Autodesk Inventor part; units mm, degrees
ref_plane "YZ Plane" through (0, 0, 0) normal (1, 0, 0) x (0, 1, 0)
ref_plane "XZ Plane" through (0, 0, 0) normal (0, 1, 0) x (-1, 0, 0)
ref_plane "XY Plane" through (0, 0, 0) normal (0, 0, 1) x (1, 0, 0)
sketch "Skizze1" plane through (0, 0, 0) normal (0, 1, 0) x (-1, 0, 0)
  line L0 (0, 0) -> (-206, 0)
  line L1 (-206, 0) -> (-206, -100)
  line L2 (-206, -100) -> (0, -100)
  line L3 (0, -100) -> (0, 0)
  dimension "d0" = 206
  dimension "d1" = 100
extrude "Extrusion1" add sketch "Skizze1" along normal blind 10
sketch "Skizze2" plane through (0, 10, 0) normal (0, 1, 0) x (1, 0, 0)
  line L0 (206, 100) -> (0, 100) construction
  line L1 (0, 100) -> (0, 20) construction
  line L2 (0, 100) -> (0, 0) construction
  line L3 (0, 100) -> (80, 100) construction
  line L4 (0, 20) -> (206, 20) construction
  line L5 (206, 20) -> (103, 20) construction
  line L6 (206, 20) -> (309, 20) construction
  line L7 (103, 20) -> (153, 20) construction
  line L8 (103, 20) -> (153, 20) construction
  line L9 (153, 20) -> (147, 20)
  line L10 (147, 20) -> (147, 26)
  line L11 (147, 26) -> (153, 26)
  line L12 (153, 26) -> (153, 20)
  line L13 (147, 20) -> (153, 20)
  line L14 (153, 20) -> (153, 14)
  line L15 (153, 14) -> (147, 14)
  line L16 (147, 14) -> (147, 20)
  arc A0 (147, 14) -> (153, 8) centre (153, 14) ccw
  arc A1 (153, 32) -> (147, 26) centre (153, 26) ccw
  line L17 (153, 8) -> (153, 32)
  line L18 (306, 20) -> (100, 20) construction
  line L19 (100, 20) -> (203, 20) construction
  line L20 (203, 20) -> (153, 20) construction
  line L21 (203, 20) -> (153, 20) construction
  line L22 (153, 20) -> (159, 20)
  line L23 (159, 20) -> (159, 26)
  line L24 (159, 26) -> (153, 26)
  line L25 (159, 20) -> (153, 20)
  line L26 (153, 14) -> (159, 14)
  line L27 (159, 14) -> (159, 20)
  arc A2 (153, 8) -> (159, 14) centre (153, 14) ccw
  arc A3 (159, 26) -> (153, 32) centre (153, 26) ccw
  line L28 (103, 100) -> (103, 20) construction
  line L29 (0, 0) -> (206, 0) construction
  line L30 (103, 100) -> (183, 100) construction
  line L31 (53, 20) -> (59, 20)
  line L32 (59, 20) -> (59, 26)
  line L33 (59, 26) -> (53, 26)
  line L34 (53, 26) -> (53, 20)
  line L35 (59, 20) -> (53, 20)
  line L36 (53, 20) -> (53, 14)
  line L37 (53, 14) -> (59, 14)
  line L38 (59, 14) -> (59, 20)
  arc A4 (53, 8) -> (59, 14) centre (53, 14) ccw
  arc A5 (59, 26) -> (53, 32) centre (53, 26) ccw
  line L39 (53, 8) -> (53, 32)
  line L40 (47, 20) -> (47, 26)
  line L41 (47, 26) -> (53, 26)
  line L42 (53, 20) -> (47, 20)
  line L43 (47, 20) -> (53, 20)
  line L44 (47, 14) -> (47, 20)
  line L45 (53, 14) -> (47, 14)
  arc A6 (53, 32) -> (47, 26) centre (53, 26) ccw
  arc A7 (47, 14) -> (53, 8) centre (53, 14) ccw
  dimension "d4" = 80
  dimension "d5" = 90
  dimension "d6" = 206
  dimension "d7" = 90
  dimension "d8" = 103
  dimension "d9" = 180
  dimension "d10" = 50
  dimension "d11" = 0
  dimension "d12" = 6
  dimension "d13" = 6
  dimension "d14" = 6
  dimension "d15" = 6
  dimension "d16" = 80
  dimension "d17" = 90
extrude "Extrusion2" cut sketch "Skizze2" against normal blind 10
sketch "Skizze4" plane through (0, 10, 0) normal (0, 1, 0) x (1, 0, 0)
  line L0 (0, 100) -> (0, 80) construction
  line L1 (0, 100) -> (0, 0) construction
  line L2 (0, 100) -> (20, 100) construction
  line L3 (0, 80) -> (206, 80) construction
  line L4 (0, 80) -> (103, 80) construction
  line L5 (103, 80) -> (53, 80) construction
  line L6 (53, 80) -> (153, 80) construction
  dimension "d24" = 20
  dimension "d25" = 90
  dimension "d26" = 206
  dimension "d27" = 90
  dimension "d28" = 50
  dimension "d29" = 100
  dimension "d30" = 0
hole "Bohrung1" at (153, 10, -80) at (53, 10, -80) direction (0, -1, 0) diameter 11 end through all countersink diameter 20 countersink angle 90
properties part number "Motorhalterung_BT1"
For this review, take the finished solid that the model builds, in its own axes (mm). A direction names the side the tool comes from. Coordinates: 2 decimals unless noted, no trailing zeros. Loops run counter-clockwise (first coordinate to the right, second up) from the corner with the lowest first, then second, coordinate; pieces in that order, holes last. Notation, with made-up numbers: (79, 14) -> (136, 14) arc R17 ccw to (136, 38) -> close; hole circle Ø3 at (-32, 0.25). An arc over 180 degrees is marked (long way). Write each question's results on one line, items separated by ' | '.
Q1. To check wall thickness, follow line 1 along X through (y, z) = (6.5, -26); line 2 along X through (y, z) = (1.95, -80); line 3 along Z through (x, y) = (153, 2.15). State the ranges of each line that lie inside material, in increasing order. Write a range as [from, to].
Taken from the geometry:
line 1: [0, 47], [59, 147], [159, 206] | line 2: [0, 47.5], [58.5, 147.5], [158.5, 206] | line 3: [-100, -85.5], [-74.5, -32], [-8, 0]
Q2. For pin 1 Ø10 at (x, z) = (153, -80) entering from -Y, flat-tipped, find the tip position at first contact; note if it passes through.
Taken from the geometry:
pin 1: through
Q3. Machinability: for faces 1 (the cylindrical face through (53, 5, -8)), 2 (the flat face through (104, 0, -49)), which of the approach directions +Z, -Z, +X, -X, +Y, -Y give a long, thin tool a straight path to every point of the face, cutting with its end or side? Answer none if there is none.
Taken from the geometry:
face 1: +Y, -Y | face 2: +Z, -Z, +X, -X, -Y
Q4. Add section A-A, the plane z = -80. State the section outline as (x, y) points, then the cut area to 3 significant figures.
Taken from the geometry:
outline: (0, 0) -> (47.5, 0) -> (47.5, 5.5) -> (43, 10) -> (0, 10) -> close; (58.5, 0) -> (147.5, 0) -> (147.5, 5.5) -> (143, 10) -> (63, 10) -> (58.5, 5.5) -> close; (158.5, 0) -> (206, 0) -> (206, 10) -> (163, 10) -> (158.5, 5.5) -> close | area: 1,800 mm²
Q5. Mouldability with a two-part tool opening along Z and no side actions: class faces 3 (the flat face through (102, 5, 0)), 4 (the flat face through (147, 5, -20)), 5 (the flat face through (104, 5, -100)) as +Z half, -Z half, draft (parallel to the pull), parting line (faces both ways), or undercut.
Taken from the geometry:
face 3: +Z half | face 4: undercut | face 5: -Z half
Q6. Add section C-C, the plane x = 53. State the section outline as (y, z) points, then the cut area to 3 significant figures.
Taken from the geometry:
outline: (0, -100) -> (10, -100) -> (10, -90) -> (5.5, -85.5) -> (0, -85.5) -> close; (0, -74.5) -> (5.5, -74.5) -> (10, -70) -> (10, -32) -> (0, -32) -> close; (0, -8) -> (10, -8) -> (10, 0) -> (0, 0) -> close | area: 630 mm²
Q7. Add section B-B, the plane y = 2.25. State the section outline as (x, z) points.
Taken from the geometry:
outline: (0, -100) -> (206, -100) -> (206, 0) -> (0, 0) -> close; hole (47, -26) arc R6 ccw to (59, -26) -> (59, -14) arc R6 ccw to (47, -14) -> close; hole circle Ø11 at (53, -80); hole (147, -26) arc R6 ccw to (159, -26) -> (159, -14) arc R6 ccw to (147, -14) -> close; hole circle Ø11 at (153, -80)
